Input: dimensioned drawing with shaded views. Units: mm. Origin: part minimum x, y, z. A direction names the side the tool comes from. Coordinates: 2 decimals unless noted, no trailing zeros. Loops run counter-clockwise (first coordinate to the right, second up) from the corner with the lowest first, then second, coordinate; pieces in that order, holes last.
Item 1: Section B-B on x = 179. Return loops of the section in (y, z), and give its area (3 significant figures).
Item 2: Reachability of the marked faces 4, 5 and 6 from +Z, -Z, +X, -X, +Y, -Y: full face, straight path, thin tool, end or side. Return the list, or none.
Item 3: Section D-D on x = 83.5. Return loops of the section in (y, z), and give its area (3 significant figures).
Item 4: Ray query, line 1 along Y through (x, z) = (0.95, 150); line 2 along Z through (x, y) = (102, 46.55); line 3 along Y through (x, z) = (22.5, 115.5). Return the intervals inside material, ascending.
Item 5: Section A-A on y = 28.5. Return loops of the section in (x, z).
Item 6: Pull-direction query (X, two-part tool) for the marked faces 1, 2 and 3; classes: released by +X, released by -X, zero draft, split by the parting line, or undercut.
Item 7: Section C-C on z = 36.5. Return loops of the section in (x, y), and give its area (3 significant figures).
Item 8: Contact query for flat-ended pins moving along their axis: P1, Ø6.5, axis at x = 102, z = 12.52, coming from the -Y side; P2, Ø16, axis at y = 31.5, z = 148, coming from the -X side. Output: stop coordinate, or through.
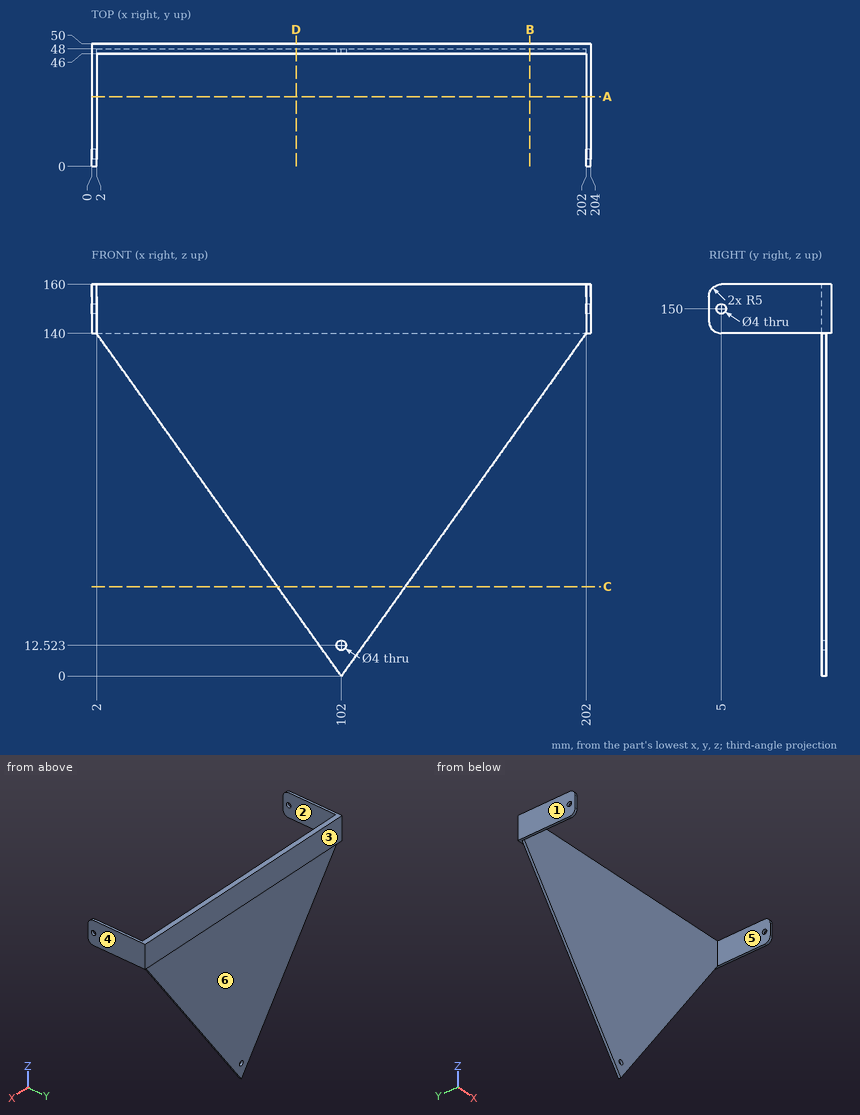
Results found:
1. outline: (46, 107.8) - (48, 107.8) - (48, 140) - (50, 140) - (50, 160) - (46, 160) - close
1. area: 144 mm2
2. face 4: +Z, -Z, +X, +Y, -Y
2. face 5: +Z, -Z, -Y
2. face 6: -Z, +X, -X, +Y
3. outline: (46, 25.9) - (48, 25.9) - (48, 140) - (50, 140) - (50, 160) - (46, 160) - close
3. area: 308 mm2
4. line 1: y = 0 to 3, 7 to 50
4. line 2: z = 0 to 10.52, 14.52 to 160
4. line 3: y = 46 to 48
5. outline: (0, 140) - (2, 140) - (2, 160) - (0, 160) - close; (202, 140) - (204, 140) - (204, 160) - (202, 160) - close
6. face 1: released by -X
6. face 2: undercut
6. face 3: zero draft
7. outline: (75.93, 46) - (128.07, 46) - (128.07, 48) - (75.93, 48) - close
7. area: 104 mm2
8. P1: stops at y = 46
8. P2: stops at x = 0
